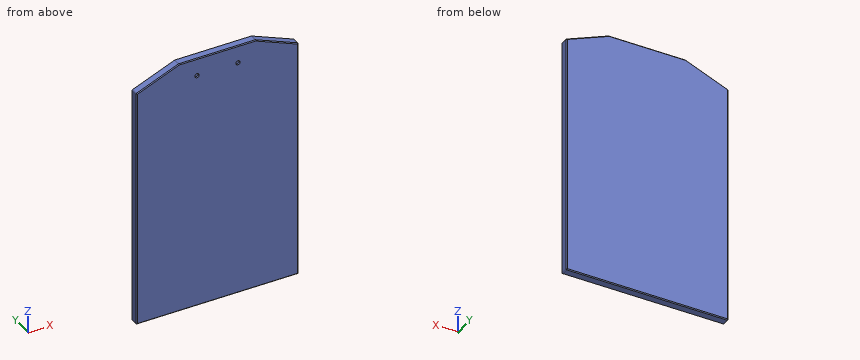
from build123d import *

# Parameters (mm, degrees)
F1_DEPTH = 12.7
F2_SIZE  = 1.27
F3_R     = 1.27
F5_DEPTH = 2.54


with BuildPart() as f1:
    # F0 (on Front) → F1 (new body)
    with BuildSketch(Plane.XZ):
        Polygon((-120.65, -190.5), (120.65, -190.5), (120.65, 165.1), (57.15, 190.5), (-57.15, 190.5), (-120.65, 165.1), align=None)
    extrude(amount=F1_DEPTH)

    # F2
    f2_edges = [f1.edges().sort_by_distance(p)[0] for p in [
        (-88.9, -12.7, 177.8),
        (0, -12.7, 190.5),
        (88.9, -12.7, 177.8),
        (120.65, -12.7, -12.7),
        (0, -12.7, -190.5),
        (-120.65, -12.7, -12.7),
        (120.65, 0, -12.7),
        (0, 0, -190.5),
        (-120.65, 0, -12.7),
        (-88.9, 0, 177.8),
        (0, 0, 190.5),
        (88.9, 0, 177.8),
    ]]
    chamfer(f2_edges, length=F2_SIZE)

    # F3
    f3_edges = [f1.edges().sort_by_distance(p)[0] for p in [
        (-120.65, -6.35, 165.1),
        (-57.15, -6.35, 190.5),
        (57.15, -6.35, 190.5),
        (120.65, -6.35, 165.1),
        (120.65, -6.35, -190.5),
        (-120.65, -6.35, -190.5),
    ]]
    fillet(f3_edges, radius=F3_R)

    # F4 (on face) → F5 (cut)
    with BuildSketch(Plane.XZ.offset(12.7)):
        with BuildLine():
            ThreePointArc((27.305, 164.240168139), (30.48, 161.065168139), (33.655, 164.240168139))
            Line((33.655, 164.240168139), (27.305, 164.240168139))
        make_face()
        with BuildLine():
            Line((27.305, 164.240168139), (33.655, 164.240168139))
            ThreePointArc((33.655, 164.240168139), (30.48, 167.415168139), (27.305, 164.240168139))
        make_face()
        with BuildLine():
            Line((-33.655, 164.240168139), (-27.305, 164.240168139))
            ThreePointArc((-27.305, 164.240168139), (-30.48, 167.415168139), (-33.655, 164.240168139))
        make_face()
        with BuildLine():
            ThreePointArc((-33.655, 164.240168139), (-30.48, 161.065168139), (-27.305, 164.240168139))
            Line((-27.305, 164.240168139), (-33.655, 164.240168139))
        make_face()
    extrude(amount=-F5_DEPTH, mode=Mode.SUBTRACT)


solid = f1.part
Geometry: final body of the model. Coordinates: model frame, mm. Coordinates: 2 decimals unless noted, no trailing zeros. Order: outer loops, then holes, each group sorted by start corner. A loop starts at its lowest first (then second) coordinate and runs counter-clockwise, first axis right, second up.
1) First-contact query: P1, Ø8.5, axis at x = -30.48, z = 164.24, coming from the -Y side; P2, Ø3, axis at x = 29.5, z = 165, coming from the -Y side; P3, Ø6, axis at x = 93.5, y = -6, coming from the +Z side. Flat tips, straight axial feed; report the tip coordinate or a pass-through.
Result sheet:
P1: stops at y = -12.7
P2: stops at y = -10.16
P3: stops at z = 177.16
2) Section B-B (x = 99). Return loops of the section in (y, z).
Result sheet:
outline: (-12.7, -189.23) - (-11.43, -190.5) - (-1.27, -190.5) - (0, -189.23) - (0, 172.39) - (-1.27, 173.76) - (-11.43, 173.76) - (-12.7, 172.39) - close
3) Section A-A (y = -5.75). Return loops of the section in (x, z), then the cut area to 3 significant figures.
Result sheet:
outline: (-120.65, -189.23) arc R1.27 ccw to (-119.38, -190.5) - (119.38, -190.5) arc R1.27 ccw to (120.65, -189.23) - (120.65, 164.24) arc R1.27 ccw to (119.85, 165.42) - (57.38, 190.41) arc R1.27 ccw to (56.91, 190.5) - (-56.91, 190.5) arc R1.27 ccw to (-57.38, 190.41) - (-119.85, 165.42) arc R1.27 ccw to (-120.65, 164.24) - close
area: 90,300 mm2
4) Ray query, probe 1 along Z at (x, y) = (-30.48, -11.2); probe 2 along Z at (x, y) = (-30.48, -12.1); probe 3 along X at (y, z) = (-1, 4.5). Return the intervals inside material, ascending.
Result sheet:
probe 1: z = -190.5 to 161.07, 167.42 to 190.5
probe 2: z = -189.83 to 161.07, 167.42 to 189.83
probe 3: x = -120.38 to 120.38
